```python
from build123d import *

# Parameters (mm, degrees)
SALIENTE_EXTRUIR2_DEPTH = 8
CROQUIS3_R              = 0.5
CORTAR_EXTRUIR1_DEPTH   = 45
REDONDEO1_R             = 1
REDONDEO2_R             = 1
REDONDEO3_R             = 1
REDONDEO4_R             = 1


with BuildPart() as part:
    # Croquis1 → Saliente-Extruir2 (new body)
    with BuildSketch(Plane.XY):
        Polygon((0, 0), (5, 0), (5, 7), (11, 7), (11, 0), (29, 0), (29, 7), (35, 7), (35, 0), (40, 0), (40, 25), (35.5, 25), (35.5, 18), (29.5, 18), (29.5, 25), (11, 25), (11, 18), (5, 18), (5, 25), (0, 25), align=None)
    extrude(amount=SALIENTE_EXTRUIR2_DEPTH)

    # Croquis3 → Cortar-Extruir1 (cut)
    with BuildSketch(Plane(origin=(40, 0, 0), x_dir=(0, 0, -1), z_dir=(1, 0, 0))):
        with Locations((-4, 23.498247599)):
            Circle(CROQUIS3_R)
        with Locations((-4, 1.501752401)):
            Circle(CROQUIS3_R)
    extrude(amount=-CORTAR_EXTRUIR1_DEPTH, mode=Mode.SUBTRACT)

    # Redondeo1
    redondeo1_edges = [part.edges().sort_by_distance(p)[0] for p in [
        (20, 0, 8),
    ]]
    fillet(redondeo1_edges, radius=REDONDEO1_R)

    # Redondeo2
    redondeo2_edges = [part.edges().sort_by_distance(p)[0] for p in [
        (37.5, 0, 8),
        (40, 12.5, 8),
        (37.75, 25, 8),
    ]]
    fillet(redondeo2_edges, radius=REDONDEO2_R)

    # Redondeo3
    redondeo3_edges = [part.edges().sort_by_distance(p)[0] for p in [
        (20.25, 25, 8),
    ]]
    fillet(redondeo3_edges, radius=REDONDEO3_R)

    # Redondeo4
    redondeo4_edges = [part.edges().sort_by_distance(p)[0] for p in [
        (0, 12.5, 8),
        (2.5, 25, 8),
        (2.5, 0, 8),
    ]]
    fillet(redondeo4_edges, radius=REDONDEO4_R)


solid = part.part
```
Source: CAD feature listing. Evaluate the final solid. Frame: model axes, mm. A direction names the side the tool comes from. Coordinates: 2 decimals unless noted, no trailing zeros. Order: outer loops, then holes, each group sorted by start corner. A loop starts at its lowest first (then second) coordinate and runs counter-clockwise, first axis right, second up. Notation, with made-up numbers: (24.5, -16.5) - (70.5, -16.5) arc R23 cw to (70.5, 13.5) - close; hole circle Ø10 at (-15, -2.5). An arc over 180 degrees is marked (long way). One line per item, written item: value.
1) Mould query, pull axis X, two halves, no side actions, for faces 1 (the face through (11, 22, 4)), 2 (the face through (40, 12, 3)), 3 (the face through (20, 13, 0)), 4 (the face through (5, 3, 4)). Classes: released by +X, released by -X, zero draft, split by the parting line, or undercut.
Computed values:
face 1: undercut
face 2: released by +X
face 3: zero draft
face 4: undercut
2) Reachability of faces 5 (the face through (37, 0, 3)), 6 (the face through (32, 7, 4)), 7 (the face through (33, 18, 4)) from +Z, -Z, +X, -X, +Y, -Y: full face, straight path, thin tool, end or side. Return the list, or none.
Computed values:
face 5: +Z, -Z, +X, -X, -Y
face 6: +Z, -Z, -Y
face 7: +Z, -Z, +Y
3) Cut plane B-B on z = 1.75. Output: boundary loops of the cut face in (x, y).
Computed values:
outline: (0, 0) - (5, 0) - (5, 7) - (11, 7) - (11, 0) - (29, 0) - (29, 7) - (35, 7) - (35, 0) - (40, 0) - (40, 25) - (35.5, 25) - (35.5, 18) - (29.5, 18) - (29.5, 25) - (11, 25) - (11, 18) - (5, 18) - (5, 25) - (0, 25) - close
4) Ray query, line 1 (Y direction, x = 2.85, z = 4); line 2 (X direction, y = 6, z = 0.75); line 3 (X direction, y = 22, z = 2.25). Return the intervals inside material, ascending. Write a range as [from, to].
Computed values:
line 1: y = [0, 1], [2, 23], [24, 25]
line 2: x = [0, 5], [11, 29], [35, 40]
line 3: x = [0, 5], [11, 29.5], [35.5, 40]
5) Cut plane A-A on y = 22.25. Output: boundary loops of the cut face in (x, z).
Computed values:
outline: (0, 0) - (5, 0) - (5, 8) - (1, 8) arc R1 ccw to (0, 7) - close; (11, 0) - (29.5, 0) - (29.5, 8) - (11, 8) - close; (35.5, 0) - (40, 0) - (40, 7) arc R1 ccw to (39, 8) - (35.5, 8) - close
6) Cut plane C-C on z = 4. State how many separate pieces and enclosed holes the cut face has, plus the area to 3 significant figures.
Computed values:
separate pieces: 7
enclosed holes: 0
area: 776 mm^2
7) Cut plane D-D on x = 31.5. Output: boundary loops of the cut face in (y, z).
Computed values:
outline: (7, 0) - (18, 0) - (18, 8) - (7, 8) - close
8) Contact query for a flat-ended pin moving along its axis: pin 1 (1.8 mm diameter, centred on x = 7, z = 4.5, fed in from +Y). Output: stop coordinate, or through.
Computed values:
pin 1: stops at y = 18
